Input: part model. Units: mm. Frame: model coordinates. Face numbers are marked on the shaded views. A direction names the side the tool comes from. Coordinates: 2 decimals unless noted, no trailing zeros. Order: outer loops, then holes, each group sorted by start corner. A loop starts at its lowest first (then second) coordinate and runs counter-clockwise, first axis right, second up. Notation, with made-up numbers: (-14.5, 67.5) - (39.5, 67.5) arc R19 cw to (39.5, 98.5) - close; hole circle Ø3 at (-31, -10.75). An arc over 180 degrees is marked (long way). One line per question, with ' | ' between items. Start each with the question number.
```python
from build123d import *

# Parameters (mm, degrees)
F0_R     = 2.15
F0_W     = 17
F0_H     = 2
F0_W_2   = 23
F1_DEPTH = 5
F2_R     = 2.65
F3_DEPTH = 3.8
F3_TAPER = 1.5
F4_D     = 3.5
F5_R     = 2.5


with BuildPart() as f1:
    # F0 (on Right) → F1 (new body)
    with BuildSketch(Plane.YZ):
        Polygon((-20, -20), (20, -20), (20, 20), (3, 20), (-20, 20), align=None)
        with Locations((-16, -16)):
            Circle(F0_R, mode=Mode.SUBTRACT)
        with Locations((16, -16)):
            Circle(F0_R, mode=Mode.SUBTRACT)
        with BuildLine():
            Line((11.85, 16.5), (11.85, 16))
            ThreePointArc((11.85, 16), (13.0655068581, 13.0655068581), (16, 11.85))
            Line((16, 11.85), (16.5, 11.85))
            ThreePointArc((16.5, 11.85), (17.9142135624, 11.2642135624), (18.5, 9.85))
            Line((18.5, 9.85), (18.5, -9.85))
            ThreePointArc((18.5, -9.85), (17.9142135624, -11.2642135624), (16.5, -11.85))
            Line((16.5, -11.85), (16, -11.85))
            ThreePointArc((16, -11.85), (13.0655068581, -13.0655068581), (11.85, -16))
            Line((11.85, -16), (11.85, -16.5))
            ThreePointArc((11.85, -16.5), (11.2642135624, -17.9142135624), (9.85, -18.5))
            Line((9.85, -18.5), (-9.85, -18.5))
            ThreePointArc((-9.85, -18.5), (-11.2642135624, -17.9142135624), (-11.85, -16.5))
            Line((-11.85, -16.5), (-11.85, -16))
            ThreePointArc((-11.85, -16), (-13.0655068581, -13.0655068581), (-16, -11.85))
            Line((-16, -11.85), (-16.5, -11.85))
            ThreePointArc((-16.5, -11.85), (-17.9142135624, -11.2642135624), (-18.5, -9.85))
            Line((-18.5, -9.85), (-18.5, 9.85))
            ThreePointArc((-18.5, 9.85), (-17.9142135624, 11.2642135624), (-16.5, 11.85))
            Line((-16.5, 11.85), (-16, 11.85))
            ThreePointArc((-16, 11.85), (-13.0655068581, 13.0655068581), (-11.85, 16))
            Line((-11.85, 16), (-11.85, 16.5))
            ThreePointArc((-11.85, 16.5), (-11.2642135624, 17.9142135624), (-9.85, 18.5))
            Line((-9.85, 18.5), (9.85, 18.5))
            ThreePointArc((9.85, 18.5), (11.2642135624, 17.9142135624), (11.85, 16.5))
        make_face(mode=Mode.SUBTRACT)
        with Locations((-16, 16)):
            Circle(F0_R, mode=Mode.SUBTRACT)
        with Locations((16, 16)):
            Circle(F0_R, mode=Mode.SUBTRACT)
        with Locations((11.5, 21)):
            Rectangle(F0_W, F0_H)
        with Locations((-8.5, 21)):
            Rectangle(F0_W_2, F0_H)
        Polygon((-27, 20), (-20, 20), (-20, 22), (3, 22), (3, 28.5), (-27, 28.5), align=None)
        with Locations((-16, 16)):
            Circle(F0_R)
        with Locations((16, 16)):
            Circle(F0_R)
        with Locations((-16, -16)):
            Circle(F0_R)
        with Locations((16, -16)):
            Circle(F0_R)
    extrude(amount=F1_DEPTH)

    # F2 (on face) → F3 (cut)
    with BuildSketch(Plane.YZ.offset(5)):
        with Locations((-16, 16)):
            Circle(F2_R)
        with Locations((16, 16)):
            Circle(F2_R)
        with Locations((16, -16)):
            Circle(F2_R)
        with Locations((-16, -16)):
            Circle(F2_R)
    extrude(amount=-F3_DEPTH, taper=F3_TAPER, mode=Mode.SUBTRACT)

    # F4 (through all)
    with Locations(Plane(origin=(0, 0, 0), x_dir=(0, 1, 0), z_dir=(-1, 0, 0))):
        with Locations((-16, -16), (16, -16), (16, 16), (-16, 16)):
            Hole(F4_D / 2)

    # F5
    f5_edges = [f1.edges().sort_by_distance(p)[0] for p in [
        (2.5, 3, 22),
        (2.5, 3, 28.5),
        (2.5, 20, 22),
        (2.5, 20, -20),
        (2.5, -20, -20),
        (2.5, -20, 20),
        (2.5, -27, 20),
        (2.5, -27, 28.5),
    ]]
    fillet(f5_edges, radius=F5_R)


solid = f1.part
```
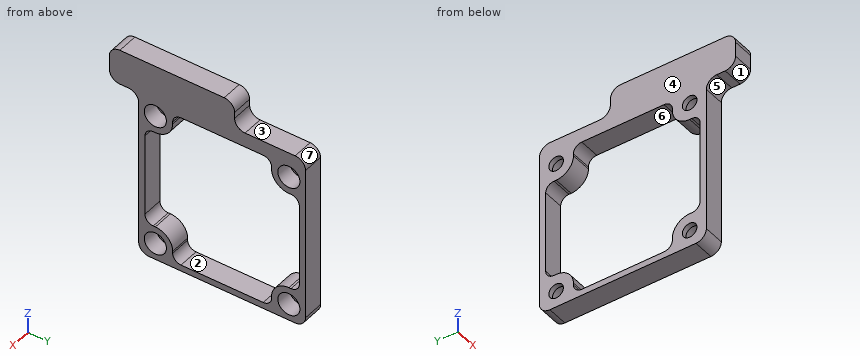
(1) Draft query along Y for the marked faces 4, 5, 6 and 7. Return one class per face: +Y half, -Y half, draft (parallel to the pull), parting line (faces both ways), or undercut.
(2) Section B-B (y = 4). Output: boundary loops of the cut face in (x, z).
(3) Section A-A (z = 9). Output: boundary loops of the cut face in (x, y), then the cut area to 3 significant figures.
(4) Material intervals for line 1 along Y through (x, z) = (0.5, -16); line 2 along Z through (x, y) = (1.05, -16), sorted ascending. Write a range as from..to.
(5) Reachability of the marked faces 1, 2 and 3 from +Z, -Z, +X, -X, +Y, -Y: full face, straight path, thin tool, end or side. Return the list, or none.
(6) Pin query (flat end, axial travel): pin 1 (3 mm diameter, centred on x = 4, z = 8.5, fed in from -Y); pin 2 (2.5 mm diameter, centred on x = 3, y = 14.5, fed in from +Z); pin 3 (4 mm diameter, centred on y = 16, z = -16, fed in from +X). Return the tip coordinate at first contact, or that it passes through.
Worked answers:
1) face 4: draft | face 5: -Y half | face 6: undercut | face 7: +Y half
2) outline: (0, -20) - (5, -20) - (5, -18.5) - (0, -18.5) - close; (0, 18.5) - (5, 18.5) - (5, 22.5) - (0, 22.5) - close
3) outline: (0, -20) - (5, -20) - (5, -18.5) - (0, -18.5) - close; (0, 18.5) - (5, 18.5) - (5, 20) - (0, 20) - close | area: 15.0 mm²
4) line 1: y = -20..-17.75, -14.25..-11.85, 11.85..14.25, 17.75..20 | line 2: z = -20..-17.75, -14.25..-11.85, 11.85..14.25, 17.75..28.5
5) face 1: -Z, +X, -X, -Y | face 2: +X, -X | face 3: +Z, +X, -X, +Y
6) pin 1: stops at y = -20 | pin 2: stops at z = 22 | pin 3: stops at x = 1.2
